Verification items for the finished model (mm, model axes). A direction names the side the tool comes from. Coordinates: 2 decimals unless noted, no trailing zeros. Loops run counter-clockwise (first coordinate to the right, second up) from the corner with the lowest first, then second, coordinate; pieces in that order, holes last. Notation, with made-up numbers: (37, 29.25) -> (81, 29.25) arc R15 ccw to (81, 38.25) -> close; hole circle Ø10 at (55.5, 48). An arc over 180 degrees is marked (long way). Answer as a JSON object with one key per item and string values. Group by question number.
Q1. Cross-section at D-D on y = -2.75. Record the boundary of the cut face in (x, z).
Q2. Gauge pin test, flat ends, axial feed: pin 1 Ø3 at (x, y) = (5.5, 3.5) entering from +Z; pin 2 Ø8 at (x, y) = (20, 4.5) entering from -Z; pin 3 Ø5 at (x, y) = (11.5, 5) entering from +Z. Record the tip position at first contact, or that the pin passes through.
Q3. Release check for a two-part mould opening along Y. For faces 1 (the flat face through (-0.2, 0, 0.5)), 2 (the flat face through (20, 4, 0.2)), 3 (the flat face through (0.6, 8.33, 0.5)), 4 (the flat face through (9.865, 2.167, 0.496)) record: released by +Y, released by -Y, zero draft, split by the parting line, or undercut.
Q4. Cross-section at A-A on y = 6. Give the number of separate pieces and of enclosed holes in the cut face, and give its area (3 significant figures).
Q5. Scan lines: L1, parallel to X at y = 8.9, z = 1.05; L2, parallel to Y at x = 16.25, z = 0.9; L3, parallel to Y at x = 15, z = 0.5. Record each from-to range of solid material in increasing order.
Q6. Cross-section at B-B on x = 15.75. Record the boundary of the cut face in (y, z).
Q7. Cross-section at C-C on y = 8.9. Record the boundary of the cut face in (x, z).
Q8. Set-up check for faces 5 (the flat face through (12.8, 9, 1)), 6 (the flat face through (0, 3.9, 0.5)), 7 (the flat face through (22.34, 5.7, 0.5)): record each of +Z, -Z, +X, -X, +Y, -Y from which the full face is reachable in a straight line by a thin tool's end or side.
```python
from build123d import *

# Parameters (mm, degrees)
SKETCH_W               = 1.25
SKETCH_H               = 8.33
PAD_DEPTH              = 1
BOX_W                  = 27.5
BOX_H                  = 0.8
BOX_DEPTH              = 1
LINEARPATTERN_COUNT    = 2
LINEARPATTERN_PITCH    = 7
BOX001_W               = 0.8
BOX001_H               = 8
BOX001_DEPTH           = 1
BOX002_W               = 0.8
BOX002_H               = 8
BOX002_DEPTH           = 1
BOX003_W               = 0.65
BOX003_H               = 14
BOX003_DEPTH           = 0.6
LINEARPATTERN001_COUNT = 2
LINEARPATTERN001_PITCH = 12.5
BOX004_W               = 0.65
BOX004_H               = 14
BOX004_DEPTH           = 0.6
LINEARPATTERN002_COUNT = 2
LINEARPATTERN002_PITCH = 13
CYLINDER_R             = 0.53
CYLINDER_DEPTH         = 12
CYLINDER001_R          = 2.8
CYLINDER001_DEPTH      = 0.4
BOX005_W               = 1.6
BOX005_H               = 1.8
BOX005_DEPTH           = 1.2
CYLINDER002_R          = 0.6
CYLINDER002_DEPTH      = 2
BOX006_W               = 4
BOX006_H               = 6
BOX006_DEPTH           = 1


with BuildPart() as part:
    # Sketch → Pad (new body)
    with BuildSketch(Plane.XY):
        with Locations((0.625, 4.165)):
            Rectangle(SKETCH_W, SKETCH_H)
    extrude(amount=PAD_DEPTH)

    # Box → Box (join)
    with BuildSketch(Plane(origin=(-0.5, 0, 0), x_dir=(1, 0, 0), z_dir=(0, 0, 1))):
        with Locations((13.75, 0.4)):
            Rectangle(BOX_W, BOX_H)
    box = extrude(amount=BOX_DEPTH)

    # LinearPattern: Box ×2
    with Locations(*[(0, i * LINEARPATTERN_PITCH, 0) for i in range(1, LINEARPATTERN_COUNT)]):
        add(box)

    # Box001 → Box001 (join)
    with BuildSketch(Plane(origin=(13.2, 0, 0), x_dir=(1, 0, 0), z_dir=(0, 0, 1))):
        with Locations((0.4, 4)):
            Rectangle(BOX001_W, BOX001_H)
    extrude(amount=BOX001_DEPTH)

    # Box002 → Box002 (join)
    with BuildSketch(Plane(origin=(26, 0, 0), x_dir=(1, 0, 0), z_dir=(0, 0, 1))):
        with Locations((0.4, 4)):
            Rectangle(BOX002_W, BOX002_H)
    extrude(amount=BOX002_DEPTH)

    # Box003 → Box003 (join)
    with BuildSketch(Plane(origin=(1, 1, 0.2), x_dir=(0.469472, -0.882948, 0), z_dir=(0, 0, 1))):
        with Locations((0.325, 7)):
            Rectangle(BOX003_W, BOX003_H)
    box003 = extrude(amount=BOX003_DEPTH)

    # LinearPattern001: Box003 ×2
    with Locations(*[(i * LINEARPATTERN001_PITCH, 0, 0) for i in range(1, LINEARPATTERN001_COUNT)]):
        add(box003)

    # Box004 → Box004 (join)
    with BuildSketch(Plane(origin=(13, 0.5, 0.2), x_dir=(0.469472, 0.882948, 0), z_dir=(0, 0, 1))):
        with Locations((0.325, 7)):
            Rectangle(BOX004_W, BOX004_H)
    box004 = extrude(amount=BOX004_DEPTH)

    # LinearPattern002: Box004 ×2
    with Locations(*[(i * LINEARPATTERN002_PITCH, 0, 0) for i in range(1, LINEARPATTERN002_COUNT)]):
        add(box004)

    # Cylinder → Cylinder (join)
    with BuildSketch(Plane(origin=(0.5, 0, 0.5), x_dir=(1, 0, 0), z_dir=(0, -1, 0))):
        Circle(CYLINDER_R)
    extrude(amount=CYLINDER_DEPTH)

    # Cylinder001 → Cylinder001 (join)
    with BuildSketch(Plane(origin=(27, 4.1, 0.6), x_dir=(1, 0, 0), z_dir=(0, 0, 1))):
        Circle(CYLINDER001_R)
    extrude(amount=CYLINDER001_DEPTH)

    # Box005 → Box005 (join)
    with BuildSketch(Plane(origin=(12.8, 7.9, 0), x_dir=(1, 0, 0), z_dir=(0, 0, 1))):
        with Locations((0.8, 0.9)):
            Rectangle(BOX005_W, BOX005_H)
    extrude(amount=BOX005_DEPTH)

    # Cylinder002 → Cylinder002 (cut)
    with BuildSketch(Plane(origin=(13.6, 8.9, 0.5), x_dir=(1, 0, 0), z_dir=(0, 0, 1))):
        Circle(CYLINDER002_R)
    extrude(amount=CYLINDER002_DEPTH, mode=Mode.SUBTRACT)

    # Box006 → Box006 (cut)
    with BuildSketch(Plane(origin=(27, 1, 0), x_dir=(1, 0, 0), z_dir=(0, 0, 1))):
        with Locations((2, 3)):
            Rectangle(BOX006_W, BOX006_H)
    extrude(amount=BOX006_DEPTH, mode=Mode.SUBTRACT)

    # Sphere → Sphere (revolve)
    with BuildSketch(Plane(origin=(13.55, 9.9, 0.6), x_dir=(1, 0, 0), z_dir=(0, -1, 0))):
        with BuildLine():
            ThreePointArc((0, -0.5), (0.5, 0), (0, 0.5))
            Line((0, 0.5), (0, -0.5))
        make_face()
    revolve(axis=Axis((13.55, 9.9, 0.6), (0, 0, 1)))


solid = part.part
```
Computed values:
{
 "1": {"outline": "circle Ø1.06 at (0.5, 0.5)"},
 "2": {"pin 1": "stops at z = 0.8", "pin 2": "stops at z = 0", "pin 3": "stops at z = 1"},
 "3": {"face 1": "released by -Y", "face 2": "undercut", "face 3": "released by +Y", "face 4": "undercut"},
 "4": {"separate pieces": "7", "enclosed holes": "0", "area": "6.68 mm²"},
 "5": {"L1": "x = 12.8 to 13, 14.2 to 14.4", "L2": "y = 0 to 0.8, 7 to 7.8", "L3": "y = 0 to 0.8, 1.06 to 1.8, 6.35 to 7.8"},
 "6": {"outline": "(0, 0) -> (0.8, 0) -> (0.8, 1) -> (0, 1) -> close; (1.46, 0.2) -> (2.2, 0.2) -> (2.2, 0.8) -> (1.46, 0.8) -> close; (5.95, 0.2) -> (6.69, 0.2) -> (6.69, 0.8) -> (5.95, 0.8) -> close; (7, 0) -> (7.8, 0) -> (7.8, 1) -> (7, 1) -> close"},
 "7": {"outline": "(12.8, 0) -> (14.4, 0) -> (14.4, 1.2) -> (14.2, 1.2) -> (14.2, 0.5) -> (13, 0.5) -> (13, 1.2) -> (12.8, 1.2) -> close"},
 "8": {"face 5": "+Z, -Z, +Y", "face 6": "+Z, -Z, -X", "face 7": "+Z, -Z"}
}
